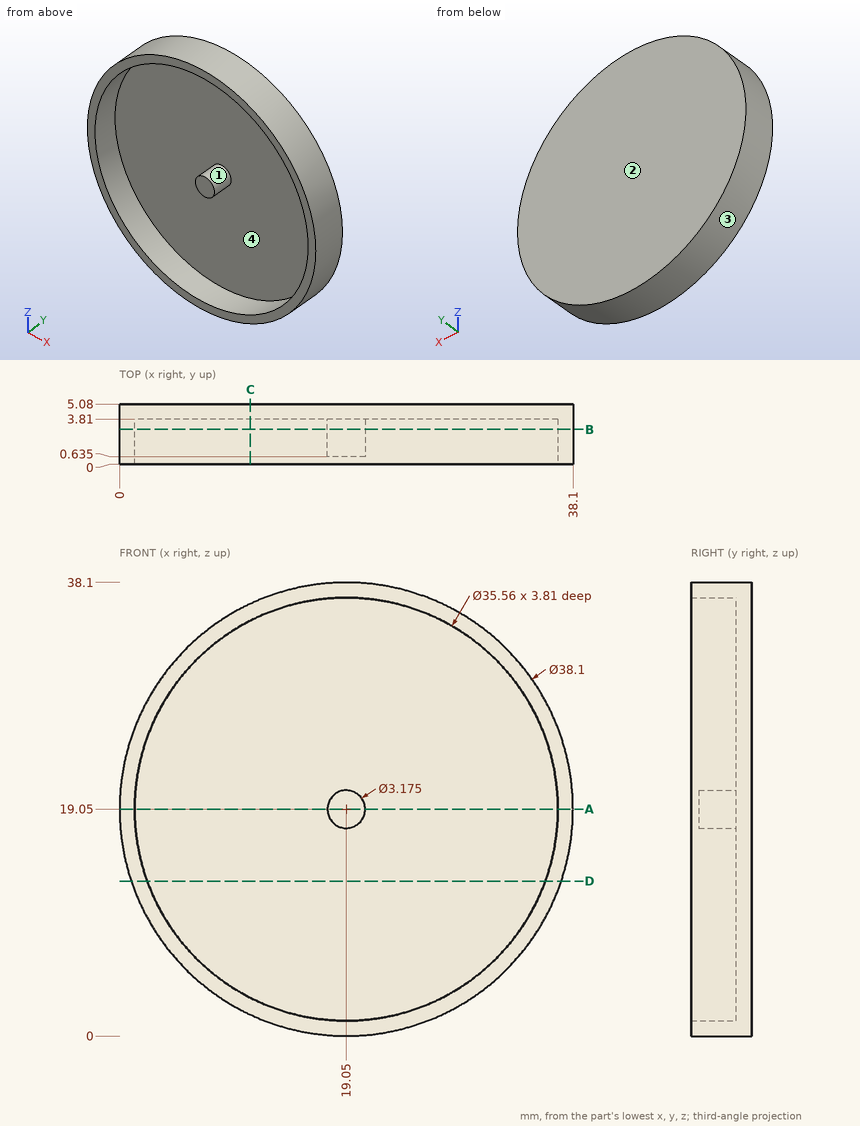
Answer from the drawing. Dimensions are ordinates in mm from the lowest x, y and z of the part. Give positions to 0.01 mm unless a question says otherwise; leave off trailing zeros. Order: outer loops, then holes, each group sorted by start corner. A loop starts at its lowest first (then second) coordinate and runs counter-clockwise, first axis right, second up. Notation, with made-up numbers: (-40, -23) - (-33, -23) arc R20 ccw to (-33, 6) - close; hole circle Ø3 at (15.5, 4.25). An arc over 180 degrees is marked (long way). Use one line per item in the form item = value.
1) Find section A-A on z = 19.05. Determine the outline of the cut face in (x, y) (1 decimal), and give its area (3 significant figures).
Verdict:
outline = (0, 0) - (1.3, 0) - (1.3, 3.8) - (17.5, 3.8) - (17.5, 0.6) - (20.6, 0.6) - (20.6, 3.8) - (36.8, 3.8) - (36.8, 0) - (38.1, 0) - (38.1, 5.1) - (0, 5.1) - close
area = 68.1 mm^2
2) Consider probe 1 along Z at (x, y) = (19.05, 0.85); probe 2 along X at (y, z) = (1.75, 18); probe 3 along Y at (x, z) = (15, 31). Determine where each line is inside the solid, lowest interval first. Write a range as [from, to].
Verdict:
probe_1 = [0, 1.27], [17.46, 20.64], [36.83, 38.1]
probe_2 = [0.03, 1.3], [17.86, 20.24], [36.8, 38.07]
probe_3 = [3.81, 5.08]
3) Find section D-D on z = 13. Determine the outline of the cut face in (x, y), and give its area (3 significant figures).
Verdict:
outline = (0.99, 0) - (2.33, 0) - (2.33, 3.81) - (35.77, 3.81) - (35.77, 0) - (37.11, 0) - (37.11, 5.08) - (0.99, 5.08) - close
area = 56.1 mm^2
4) The mould has two halves that part along Z. Classify the marked faces 1, 2, 3 and 4: released by +Z, released by -Z, zero draft, split by the parting line, or undercut.
Verdict:
face_1 = undercut
face_2 = zero draft
face_3 = split by the parting line
face_4 = undercut
5) Each of these flat-tipped pins is pushed along its axis until it touches: pin 1 (1 mm diameter, centred on x = 19.5, y = 2.5, fed in from +Z); pin 2 (1.5 mm diameter, centred on y = 1, z = 33.5, fed in from -X); pin 3 (2 mm diameter, centred on x = 33.5, y = 2, fed in from -Z). Where does it stop, or does it pass through?
Verdict:
pin_1 = 38.1
pin_2 = 5.81
pin_3 = 5.56
6) Find section C-C on x = 11. Determine the outline of the cut face in (y, z).
Verdict:
outline = (0, 1.78) - (5.08, 1.78) - (5.08, 36.32) - (0, 36.32) - (0, 34.9) - (3.81, 34.9) - (3.81, 3.2) - (0, 3.2) - close
7) Find section B-B on y = 2.95. Give the number of separate pieces and of enclosed holes in the cut face, and give its area (3 significant figures).
Verdict:
separate_pieces = 2
enclosed_holes = 1
area = 155 mm^2
